Could you check a few things on this model? Use its own coordinates, in mm. Give positions to 0.01 mm unless a question says otherwise; leave off trailing zeros. Loops run counter-clockwise (first coordinate to the right, second up) from the corner with the lowest first, then second, coordinate; pieces in that order, holes last. Notation, with made-up numbers: (43.5, 48.5) -> (54.5, 48.5) arc R24 ccw to (54.5, 79.5) -> close; hole circle Ø3 at (10.5, 15). An arc over 180 degrees is marked (long way). Write each question's results on one line, items separated by ' | '. Start each with the question number.
Q1. If I drill on line 1 along X through (y, z) = (9.5, 0); line 2 along Y through (x, z) = (-17.5, 0.1); line 3 along X through (y, z) = (15.5, -0.6), over which ranges is the centre line in solid material (lowest first)?
Q2. If we section it at C-C, the plane x = 16: List the corners of the cut face in (y, z) for me.
Q3. If we section it at A-A, the plane z = 0: List the corners of the cut face in (x, y) for me, plus the area to 3 significant figures.
Q4. If we section it at B-B, the plane y = 7: List the corners of the cut face in (x, z) for me.
from build123d import *

# Parameters (mm, degrees)
ESQUISSE2_R = 1


with BuildPart() as part:
    # Balayage1: sweep along a path in Esquisse1
    with BuildLine(Plane.XY) as balayage1_path:
        Line((-19, 23), (19, 23))
        ThreePointArc((19, 23), (20.414213562, 22.414213562), (21, 21))
        Line((21, 21), (21, -21))
        ThreePointArc((21, -21), (20.414213562, -22.414213562), (19, -23))
        Line((19, -23), (-19, -23))
        ThreePointArc((-19, -23), (-20.414213562, -22.414213562), (-21, -21))
        Line((-21, -21), (-21, 21))
        ThreePointArc((-21, 21), (-20.414213562, 22.414213562), (-19, 23))
    # Esquisse2 → Balayage1 (sweep)
    with BuildSketch(Plane(origin=(0, 0, 0), x_dir=(1, 0, 0), z_dir=(0, 1, 0))):
        with Locations((21, 0)):
            Circle(ESQUISSE2_R)
    sweep(path=balayage1_path.line)


solid = part.part
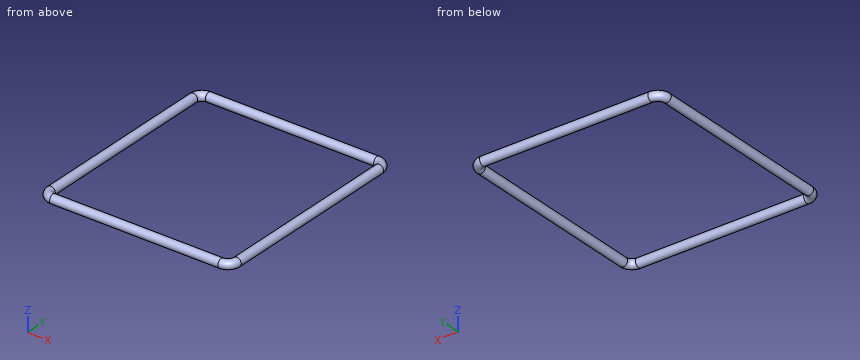
Final values:
1) line 1: x = -22 to -20, 20 to 22 | line 2: y = -23.99 to -22.01, 22.01 to 23.99 | line 3: x = -21.8 to -20.2, 20.2 to 21.8
2) outline: circle Ø2 at (-23, 0); circle Ø2 at (23, 0)
3) outline: (-22, -21) arc R3 ccw to (-19, -24) -> (19, -24) arc R3 ccw to (22, -21) -> (22, 21) arc R3 ccw to (19, 24) -> (-19, 24) arc R3 ccw to (-22, 21) -> close; hole (-20, -21) arc R1 ccw to (-19, -22) -> (19, -22) arc R1 ccw to (20, -21) -> (20, 21) arc R1 ccw to (19, 22) -> (-19, 22) arc R1 ccw to (-20, 21) -> close | area: 345 mm²
4) outline: circle Ø2 at (-21, 0); circle Ø2 at (21, 0)
